Verification items for the finished model (mm, model axes). A direction names the side the tool comes from. Coordinates: 2 decimals unless noted, no trailing zeros. Loops run counter-clockwise (first coordinate to the right, second up) from the corner with the lowest first, then second, coordinate; pieces in that order, holes last. Notation, with made-up numbers: (60, 55) -> (114, 55) arc R26 cw to (114, 93) -> close; hole circle Ø5 at (8, -10.5). An arc over 180 degrees is marked (long way). Answer as a JSON object with one key per item and string values. Group by question number.
Q1. Cross-section at C-C on y = 6.35. Record the boundary of the cut face in (x, z), and give its area (3 significant figures).
Q2. Cross-section at D-D on z = -11.5. Record the boundary of the cut face in (x, y), and give its area (3 significant figures).
Q3. Cross-section at B-B on x = 0. Record the boundary of the cut face in (y, z), and give its area (3 significant figures).
Q4. Cross-section at A-A on z = 0. Record the boundary of the cut face in (x, y), and give its area (3 significant figures).
Q5. Scan lines: L1, parallel to Z at x = 0, y = 12; L2, parallel to Y at x = -2.75, z = 6.5; L3, parallel to Z at x = -0.25, y = 6.5. Record each from-to range of solid material in increasing order.
Q6. Gauge pin test, flat ends, axial feed: pin 1 Ø1 at (y, z) = (4, -1.5) entering from +X; pin 2 Ø3 at (x, z) = (-1.5, -30.5) entering from +Y; pin 3 Ø3 at (x, y) = (4, 2) entering from +Z. Record the tip position at first contact, or that the pin passes through.
Q7. Set-up check for faces 1 (the cylindrical face through (-0.33, 12.31, -2.52)), 2 (the cylindrical face through (-0.217, 5.374, -25.496)), 3 (the flat face through (0, 0, 0)): record each of +Z, -Z, +X, -X, +Y, -Y from which the full face is reachable in a straight line by a thin tool's end or side.
```python
from build123d import *

# Parameters (mm, degrees)
SKETCH3_R           = 1
BOSS_EXTRUDE1_DEPTH = 42


with BuildPart() as part:
    # Sketch2 → Revolve1 (revolve)
    with BuildSketch(Plane.XY):
        Polygon((0, 0), (0, 12.7), (2.54, 12.7), (2.54, 11.94), (9.5, 11.94), (9.5, 0), align=None)
    revolve(axis=Axis((0, 0, 0), (0, 1, 0)))

    # Sketch3 → Boss-Extrude1 (add)
    with BuildSketch(Plane.XY):
        with Locations((0, 6.35)):
            Circle(SKETCH3_R)
    extrude(amount=-BOSS_EXTRUDE1_DEPTH)


solid = part.part
```
Computed values:
{
 "1": {"outline": "(-1, -42) -> (1, -42) -> (1, -9.45) arc R9.5 ccw (long way) to (-1, -9.45) -> close", "area": "349 mm²"},
 "2": {"outline": "circle Ø2 at (0, 6.35)", "area": "3.14 mm²"},
 "3": {"outline": "(0, -9.5) -> (5.35, -9.5) -> (5.35, -42) -> (7.35, -42) -> (7.35, -9.5) -> (11.94, -9.5) -> (11.94, -2.54) -> (12.7, -2.54) -> (12.7, 2.54) -> (11.94, 2.54) -> (11.94, 9.5) -> (0, 9.5) -> close", "area": "296 mm²"},
 "4": {"outline": "(-9.5, 0) -> (9.5, 0) -> (9.5, 11.94) -> (2.54, 11.94) -> (2.54, 12.7) -> (-2.54, 12.7) -> (-2.54, 11.94) -> (-9.5, 11.94) -> close", "area": "231 mm²"},
 "5": {"L1": "z = -2.54 to 2.54", "L2": "y = 0 to 11.94", "L3": "z = -42 to 9.5"},
 "6": {"pin 1": "stops at x = 9.45", "pin 2": "stops at y = 7.35", "pin 3": "stops at z = 9.17"},
 "7": {"face 1": "+Y", "face 2": "-Z", "face 3": "+Z, -Z, +X, -X, -Y"}
}
